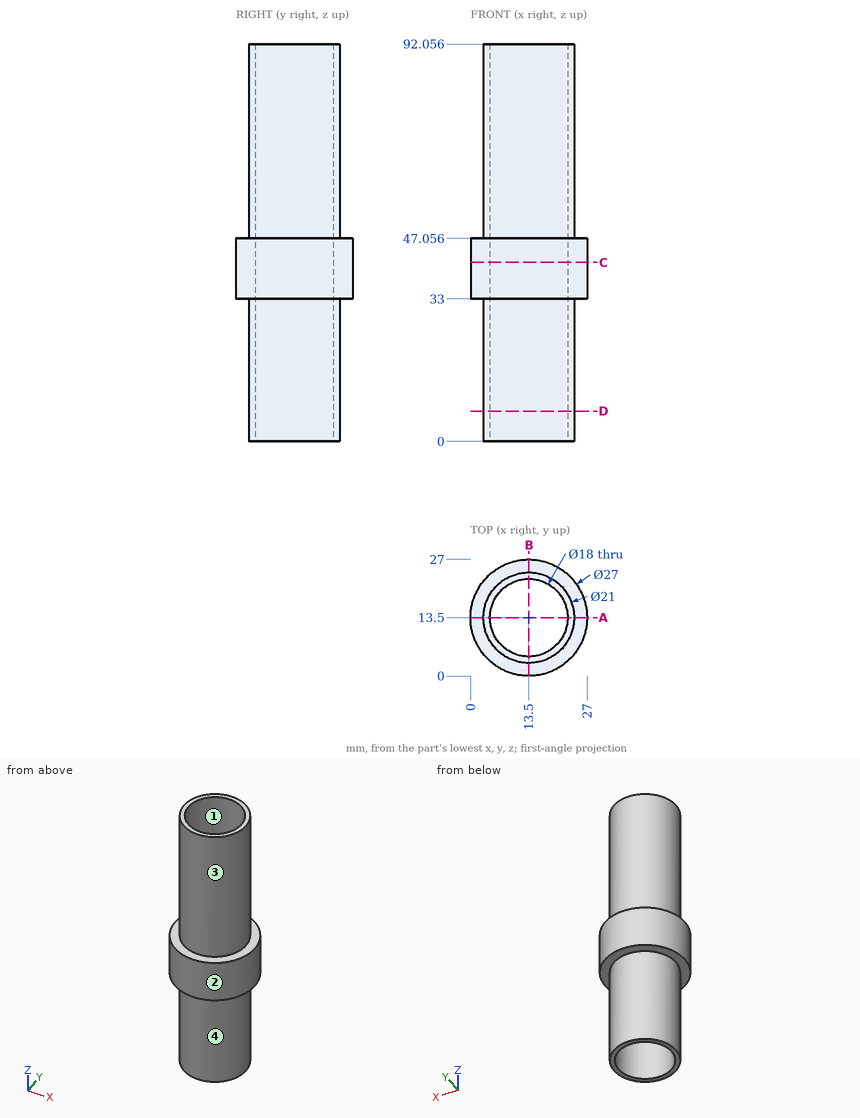
Verification items for this drawing (mm, ordinates from the low corner). A direction names the side the tool comes from. Round coordinates to 2 decimals unless told otherwise and drop trailing zeros. Order: outer loops, then holes, each group sorted by start corner. A loop starts at its lowest first (then second) coordinate and runs counter-clockwise, first axis right, second up. Notation, with made-up numbers: (0, 84.5) - (6, 84.5) arc R20 ccw to (6, 95.5) - close; hole circle Ø10 at (-7, 47.5). An arc over 180 degrees is marked (long way). Use CSV: the item, a comma, the result in double quotes.
(1) Gauge pin test, flat ends, axial feed: pin 1 Ø3 at (x, z) = (16.5, 17) entering from -Y; pin 2 Ø1 at (x, z) = (23.5, 53.5) entering from +Y; pin 3 Ø1.5 at (y, z) = (17.5, 57) entering from -X; pin 4 Ø11 at (x, y) = (13.5, 13.5) entering from +Z. Record the tip position at first contact, or that the pin passes through.
Entries:
pin 1,"y = 3.11"
pin 2,"y = 17.97"
pin 3,"x = 3.52"
pin 4,"through"
(2) Thickness scan on probe 1 along Z at (x, y) = (3.25, 19.5); probe 2 along Y at (x, z) = (13.5, 22.5); probe 3 along Y at (x, z) = (13.5, 40). Record the ranges inside material, lowest first. Write a range as from..to.
Entries:
probe 1,"33..47.06"
probe 2,"3..4.5, 22.5..24"
probe 3,"0..4.5, 22.5..27"
(3) Section check D-D on z = 7. Record the boundary of the cut face in (x, y).
Entries:
outline,"circle Ø21 at (13.5, 13.5); hole circle Ø18 at (13.5, 13.5)"
(4) Access from +Z, -Z, +X, -X, +Y, -Y to the whole of each face (thin tool, end or side, straight path). Record for the marked faces 3 and 4.
Entries:
face 3,"+Z"
face 4,"-Z"
(5) Section check A-A on y = 13.5. Record the boundary of the cut face in (x, z), and give its area (3 significant figures).
Entries:
outline,"(0, 33) - (3, 33) - (3, 0) - (4.5, 0) - (4.5, 92.06) - (3, 92.06) - (3, 47.06) - (0, 47.06) - close; (22.5, 0) - (24, 0) - (24, 33) - (27, 33) - (27, 47.06) - (24, 47.06) - (24, 92.06) - (22.5, 92.06) - close"
area,"361 mm^2"
(6) Section check C-C on z = 41.5. Record the boundary of the cut face in (x, y).
Entries:
outline,"circle Ø27 at (13.5, 13.5); hole circle Ø18 at (13.5, 13.5)"
(7) Mould release check, pull along X, two halves, no side actions. Record for the marked faces 1 and 2: released by +X, released by -X, zero draft, split by the parting line, or undercut.
Entries:
face 1,"undercut"
face 2,"split by the parting line"
